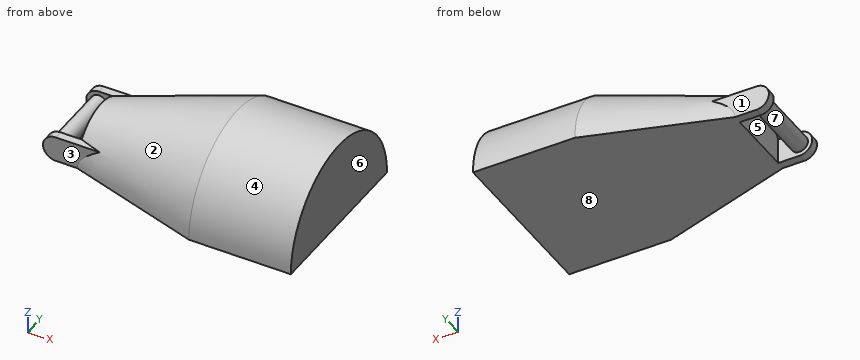
from build123d import *

# Parameters (mm, degrees)
F4_DEPTH = 19.05
F5_W     = 1.5875
F5_H     = 4.7625
F6_DEPTH = 6.35
F8_DEPTH = 25.4
F7_R     = 1.5875
F9_DEPTH = 15.875


with BuildPart() as f3:
    # F2 (on offset) → F3 section 0
    with BuildSketch(Plane.YZ.offset(-25.4)):
        with BuildLine():
            Line((-7.9375, 0), (7.9375, 0))
            ThreePointArc((7.9375, 0), (0, 7.9375), (-7.9375, 0))
        make_face()
    # F0 (on Right) → F3 section 1
    with BuildSketch(Plane.YZ):
        with BuildLine():
            ThreePointArc((15.875, 0), (0, 15.875), (-15.875, 0))
            Line((-15.875, 0), (15.875, 0))
        make_face()
    loft()

    # F4 (add): a face of the model
    f4_faces = [f3.faces().sort_by_distance(p)[0] for p in [
        (0, 0, 6.7375592576),
    ]]
    extrude(f4_faces, amount=F4_DEPTH)

    # F5 (on face) → F6 (join, symmetric)
    with BuildSketch(Plane(origin=(-25.4, 0, 0), x_dir=(0, -1, 0), z_dir=(-1, 0, 0))):
        with Locations((-7.14375, 2.38125)):
            Rectangle(F5_W, F5_H)
        with Locations((7.14375, 2.38125)):
            Rectangle(F5_W, F5_H)
    extrude(amount=F6_DEPTH, both=True)

    # F7 (on face) → F8 (cut)
    with BuildSketch(Plane(origin=(0, 7.9375, 0), x_dir=(-1, 0, 0), z_dir=(0, 1, 0))):
        with BuildLine():
            ThreePointArc((29.36875, 4.7625), (31.0525480227, 4.0650480227), (31.75, 2.38125))
            Line((31.75, 2.38125), (31.75, 4.7625))
            Line((31.75, 4.7625), (29.36875, 4.7625))
        make_face()
        with BuildLine():
            Line((31.75, 0), (31.75, 2.38125))
            ThreePointArc((31.75, 2.38125), (31.0525480227, 0.6974519773), (29.36875, 0))
            Line((29.36875, 0), (31.75, 0))
        make_face()
    extrude(amount=-F8_DEPTH, mode=Mode.SUBTRACT)

    # F7 (on face) → F9 (join)
    with BuildSketch(Plane(origin=(0, 7.9375, 0), x_dir=(-1, 0, 0), z_dir=(0, 1, 0))):
        with Locations((29.36875, 2.38125)):
            Circle(F7_R)
    extrude(amount=-F9_DEPTH)


solid = f3.part
The model under review builds one solid part; all positions refer to its coordinate system, in mm. Face numbers are marked on the shaded views. A direction names the side the tool comes from. Round coordinates to 2 decimals unless told otherwise and drop trailing zeros. Order: outer loops, then holes, each group sorted by start corner. A loop starts at its lowest first (then second) coordinate and runs counter-clockwise, first axis right, second up. Notation, with made-up numbers: (52, 42.25) -> (58, 42.25) arc R16 cw to (58, 58.25) -> close; hole circle Ø1 at (16, 77.25). An arc over 180 degrees is marked (long way). Use CSV: the item, a comma, the result in double quotes. Start each with the question number.
(1) Wall thickness on probe 1 along X at (y, z) = (-6, 1.5); probe 2 along X at (y, z) = (-7, 2.5); probe 3 along X at (y, z) = (0.5, 7): over which ranges is each line inside the solid? List them lowest first. Write a range as from..to.
(2) Mouldability with a two-part tool opening along X and no side actions: class the marked faces 6, 7 and 8 as pulls with the +X half, pulls with the -X half, needs draft (parallel to the pull), parting line crosses it, or undercut.
(3) Tool access review of the marked faces 1, 2, 3, 4 and 5: name each direction out of +Z, -Z, +X, -X, +Y, -Y from which nothing blocks a thin tool from reaching the whole face with its end or side.
(4) Insertion check: pin 1 (2 mm diameter, centred on y = 7, z = 5.5, fed in from -X); pin 2 (8.5 mm diameter, centred on y = 1, z = 3, fed in from -X); pin 3 (1.7 mm diameter, centred on x = -26.5, y = -7, fed in from +Z). Each pin has a flat end and moves straight along its axis. Give the tip position at first contact, or say it passes through.
(5) Consider section B-B on x = 9. Write out the cut boundary in (y, z) (3 decimals).
(6) Consider section C-C on x = -13. Write out the cut boundary in (y, z) (1 decimal), and give its area (3 significant figures).
Responses:
1,probe 1,"-30.69..-28.05, -25.4..19.05"
1,probe 2,"-31.75..19.05"
1,probe 3,"-25.4..19.05"
2,face 6,"pulls with the +X half"
2,face 7,"undercut"
2,face 8,"needs draft"
3,face 1,"+Z, -X, +Y"
3,face 2,"+Z, -X"
3,face 3,"+Z, -X, -Y"
3,face 4,"+Z, +X, -X"
3,face 5,"+Z, -Z"
4,pin 1,"x = -30.46"
4,pin 2,"x = -30.96"
4,pin 3,"z = 4.76"
5,outline,"(-15.875, 0) -> (15.875, 0) arc R15.875 ccw to start"
6,outline,"(-11.8, 0) -> (11.8, 0) arc R11.8 ccw to start"
6,area,"219 mm²"
